The model under review builds one solid part; all positions refer to its coordinate system, in mm. Face numbers are marked on the shaded views. Coordinates: 2 decimals unless noted, no trailing zeros. Loops run counter-clockwise (first coordinate to the right, second up) from the corner with the lowest first, then second, coordinate; pieces in that order, holes last. Notation, with made-up numbers: M 75.25,54 L 95.25,54 A21 cw 95.25,86 Z; hole C -28.75,50.25 d4. An arc over 180 degrees is marked long. Return JSON: item names as keys, results as strings.
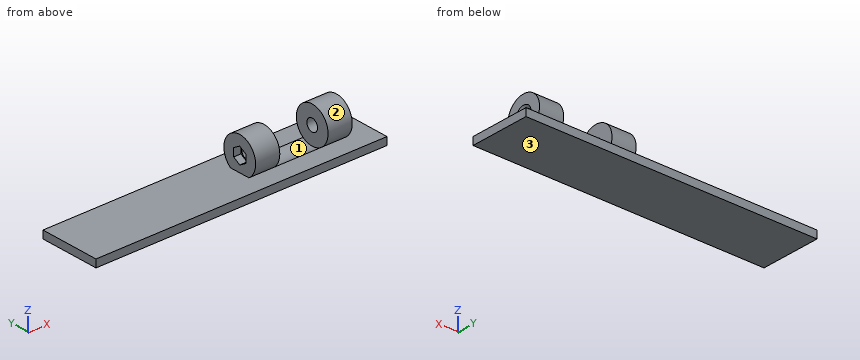
```python
from build123d import *

# Parameters (mm, degrees)
F0_W      = 120.5
F0_H      = 3.175
F1_DEPTH  = 25
F2_R      = 7.5
F3_DEPTH  = 20
F4_R      = 7.5
F5_DEPTH  = 20
F6_R      = 7.5
F7_DEPTH  = 80.5
F8_W      = 26.1427015066
F8_H      = 14.1189814121
F9_DEPTH  = 70.5
F10_W     = 25
F10_H     = 14.862489751
F11_DEPTH = 10
F12_R     = 2.5
F13_DEPTH = 80
F15_DEPTH = 3
F16_SIZE  = 1


# Not quite as in the source:
# - a feature names something its author has since deleted; it is built from what else it names


with BuildPart() as f1:
    # F0 (on Front) → F1 (new body)
    with BuildSketch(Plane.XZ):
        Rectangle(F0_W, F0_H)
    extrude(amount=F1_DEPTH)

    # F2 (on face) → F3 (join)
    with BuildSketch(Plane.YZ.offset(60.25)):
        with Locations((-12.5, 7.7303019352)):
            Circle(F2_R)
    extrude(amount=-F3_DEPTH)

    # F4 (on face) → F5 (cut)
    with BuildSketch(Plane(origin=(40.25, 0, 0), x_dir=(0, -1, 0), z_dir=(-1, 0, 0))):
        with Locations((12.5, 7.7303019352)):
            Circle(F4_R)
    extrude(amount=F5_DEPTH, mode=Mode.SUBTRACT)

    # F6 (on face) → F7 (join)
    with BuildSketch(Plane(origin=(-60.25, 0, 0), x_dir=(0, -1, 0), z_dir=(-1, 0, 0))):
        with Locations((12.5, 7.7305)):
            Circle(F6_R)
    extrude(amount=-F7_DEPTH)

    # F8 (on face) → F9 (cut)
    with BuildSketch(Plane(origin=(-60.25, 0, 0), x_dir=(0, -1, 0), z_dir=(-1, 0, 0))):
        with Locations((13.0713507533, 8.646990706)):
            Rectangle(F8_W, F8_H)
    extrude(amount=-F9_DEPTH, mode=Mode.SUBTRACT)

    # F10 (on face) → F11 (cut)
    with BuildSketch(Plane.YZ.offset(60.25)):
        with Locations((-12.5, 9.0187448755)):
            Rectangle(F10_W, F10_H)
    extrude(amount=-F11_DEPTH, mode=Mode.SUBTRACT)

    # F12 (on face) → F13 (cut)
    with BuildSketch(Plane(origin=(10.25, 0, 0), x_dir=(0, -1, 0), z_dir=(-1, 0, 0))):
        with Locations((12.5, 7.7305)):
            Circle(F12_R)
    extrude(amount=-F13_DEPTH, mode=Mode.SUBTRACT)

    # F14 (on face) → F15 (cut)
    with BuildSketch(Plane(origin=(10.25, 0, 0), x_dir=(0, -1, 0), z_dir=(-1, 0, 0))):
        Polygon((12.5147298399, 4.3905242768), (15.3998687443, 6.0732685539), (15.3851389044, 9.4132442772), (12.4852701601, 11.0704757232), (9.6001312557, 9.3877314461), (9.6148610956, 6.0477557228), align=None)
    extrude(amount=-F15_DEPTH, mode=Mode.SUBTRACT)

    # F16
    f16_edges = [f1.edges().sort_by_distance(p)[0] for p in [
        (50.25, -10, 7.7305),
    ]]
    chamfer(f16_edges, length=F16_SIZE)


solid = f1.part
```
1. The part is to be moulded in two halves that separate along Z. For the marked faces 1, 2 and 3, say which applies: released by +Z, released by -Z, zero draft, split by the parting line, or undercut.
Check values:
{"face 1": "released by +Z", "face 2": "undercut", "face 3": "released by -Z"}
2. Add section B-B on x = 41.5. Give the boundary of the cut face in (y, z), plus the area to 3 significant figures.
Check values:
{"outline": "M -25,-1.59 L 0,-1.59 L 0,1.59 L -8.2,1.59 A7.5 ccw long -16.8,1.59 L -25,1.59 Z; hole C -12.5,7.73 d5", "area": "229 mm²"}
3. Add section C-C on x = -3. Give the boundary of the cut face in (y, z), plus the area to 3 significant figures.
Check values:
{"outline": "M -25,-1.59 L 0,-1.59 L 0,1.59 L -25,1.59 Z", "area": "79.4 mm²"}
4. Add section A-A on y = -18. Give the boundary of the cut face in (x, z), plus the area to 3 significant figures.
Check values:
{"outline": "M -60.25,-1.59 L 60.25,-1.59 L 60.25,1.59 L -60.25,1.59 Z; M 10.25,2.63 L 20.25,2.63 L 20.25,12.83 L 10.25,12.83 Z; M 40.25,2.63 L 50.25,2.63 L 50.25,12.83 L 40.25,12.83 Z", "area": "587 mm²"}
5. Insertion check: pin 1 Ø4.5 at (y, z) = (-10, 8) entering from +X; pin 2 Ø6.5 at (y, z) = (-13.5, 8) entering from -X; pin 3 Ø6 at (y, z) = (-12.5, 7.73) entering from +X. Each pin has a flat end and moves straight along its axis. Give the tip position at first contact, or say it passes through.
Check values:
{"pin 1": "x = 50.25", "pin 2": "x = 10.25", "pin 3": "x = 49.75"}
6. To check wall thickness, follow line 1 (Z direction, x = 17, y = -12.5); line 2 (X direction, y = -7.5, z = 8.5); line 3 (Z direction, x = -7, y = -23). State the ranges of each line that lie inside material, in increasing order.
Check values:
{"line 1": "-1.59 to 5.23, 10.23 to 15.23", "line 2": "10.25 to 20.25, 40.25 to 50.25", "line 3": "-1.59 to 1.59"}
